```python
from build123d import *

# Parameters (mm, degrees)
F0_R     = 3
F1_DEPTH = 5
F2_R     = 3
F3_DEPTH = 3.5


with BuildPart() as f1:
    # F0 (on Top) → F1 (new body)
    with BuildSketch(Plane.XY):
        with BuildLine():
            ThreePointArc((-6.4258986346, 6.3014146616), (-5.2900672706, 7.2811529494), (-4.0072895936, 8.0586369886))
            ThreePointArc((-4.0072895936, 8.0586369886), (-6.1717451491, 8.4946784409), (-6.4258986346, 6.3014146616))
        make_face()
        with BuildLine():
            ThreePointArc((-1.4947825929, 8.875), (0, 9), (1.4947825929, 8.875))
            ThreePointArc((1.4947825929, 8.875), (1.4986950806, 8.937445581), (1.5, 9))
            ThreePointArc((1.5, 9), (-0.062554419, 10.4986950806), (-1.4947825929, 8.875))
        make_face()
        with BuildLine():
            ThreePointArc((4.0072895936, 8.0586369886), (5.2900672706, 7.2811529494), (6.4258986346, 6.3014146616))
            ThreePointArc((6.4258986346, 6.3014146616), (6.6960806145, 6.7585379123), (6.7900672706, 7.2811529494))
            ThreePointArc((6.7900672706, 7.2811529494), (5.6936967321, 8.7258270503), (4.0072895936, 8.0586369886))
        make_face()
        with BuildLine():
            ThreePointArc((7.978713358, 4.1641485505), (8.5595086467, 2.7811529494), (8.9025398062, 1.3209030997))
            ThreePointArc((8.9025398062, 1.3209030997), (9.7352098713, 1.8496344953), (10.0595086467, 2.7811529494))
            ThreePointArc((10.0595086467, 2.7811529494), (9.3898119247, 4.0303913039), (7.978713358, 4.1641485505))
        make_face()
        with BuildLine():
            ThreePointArc((10.0595086467, -2.7811529494), (9.7352098713, -1.8496344953), (8.9025398062, -1.3209030997))
            ThreePointArc((8.9025398062, -1.3209030997), (8.5595086467, -2.7811529494), (7.978713358, -4.1641485505))
            ThreePointArc((7.978713358, -4.1641485505), (9.3898119247, -4.0303913039), (10.0595086467, -2.7811529494))
        make_face()
        with BuildLine():
            ThreePointArc((6.7900672706, -7.2811529494), (6.6960806145, -6.7585379123), (6.4258986346, -6.3014146616))
            ThreePointArc((6.4258986346, -6.3014146616), (5.2900672706, -7.2811529494), (4.0072895936, -8.0586369886))
            ThreePointArc((4.0072895936, -8.0586369886), (5.6936967321, -8.7258270503), (6.7900672706, -7.2811529494))
        make_face()
        with BuildLine():
            ThreePointArc((1.5, -9), (1.4986950806, -8.937445581), (1.4947825929, -8.875))
            ThreePointArc((1.4947825929, -8.875), (0, -9), (-1.4947825929, -8.875))
            ThreePointArc((-1.4947825929, -8.875), (-0.062554419, -10.4986950806), (1.5, -9))
        make_face()
        with BuildLine():
            ThreePointArc((-6.4258986346, -6.3014146616), (-6.1717451491, -8.4946784409), (-4.0072895936, -8.0586369886))
            ThreePointArc((-4.0072895936, -8.0586369886), (-5.2900672706, -7.2811529494), (-6.4258986346, -6.3014146616))
        make_face()
        with BuildLine():
            ThreePointArc((-8.9025398062, -1.3209030997), (-9.9860934211, -3.2446784409), (-7.978713358, -4.1641485505))
            ThreePointArc((-7.978713358, -4.1641485505), (-8.5595086467, -2.7811529494), (-8.9025398062, -1.3209030997))
        make_face()
        with BuildLine():
            ThreePointArc((-8.9025398062, 1.3209030997), (-8.5595086467, 2.7811529494), (-7.978713358, 4.1641485505))
            ThreePointArc((-7.978713358, 4.1641485505), (-9.9860934211, 3.2446784409), (-8.9025398062, 1.3209030997))
        make_face()
        with BuildLine():
            ThreePointArc((8.9025398062, -1.3209030997), (8.9756018811, -0.6622468362), (9, 0))
            ThreePointArc((9, 0), (8.9756018811, 0.6622468362), (8.9025398062, 1.3209030997))
            ThreePointArc((8.9025398062, 1.3209030997), (7.1329238722, 2.3176274578), (7.978713358, 4.1641485505))
            ThreePointArc((7.978713358, 4.1641485505), (7.2811529494, 5.2900672706), (6.4258986346, 6.3014146616))
            ThreePointArc((6.4258986346, 6.3014146616), (4.4083893922, 6.0676274578), (4.0072895936, 8.0586369886))
            ThreePointArc((4.0072895936, 8.0586369886), (2.7811529494, 8.5595086467), (1.4947825929, 8.875))
            ThreePointArc((1.4947825929, 8.875), (0, 7.5), (-1.4947825929, 8.875))
            ThreePointArc((-1.4947825929, 8.875), (-2.7811529494, 8.5595086467), (-4.0072895936, 8.0586369886))
            ThreePointArc((-4.0072895936, 8.0586369886), (-3.8453931697, 7.6847824109), (-3.7900672706, 7.2811529494))
            ThreePointArc((-3.7900672706, 7.2811529494), (-4.7674522335, 5.8751396056), (-6.4258986346, 6.3014146616))
            ThreePointArc((-6.4258986346, 6.3014146616), (-7.2811529494, 5.2900672706), (-7.978713358, 4.1641485505))
            ThreePointArc((-7.978713358, 4.1641485505), (-7.3102702921, 3.6114562274), (-7.0595086467, 2.7811529494))
            ThreePointArc((-7.0595086467, 2.7811529494), (-7.6279901926, 1.6054517247), (-8.9025398062, 1.3209030997))
            ThreePointArc((-8.9025398062, 1.3209030997), (-9, 0), (-8.9025398062, -1.3209030997))
            ThreePointArc((-8.9025398062, -1.3209030997), (-7.6279901926, -1.6054517247), (-7.0595086467, -2.7811529494))
            ThreePointArc((-7.0595086467, -2.7811529494), (-7.3102702921, -3.6114562274), (-7.978713358, -4.1641485505))
            ThreePointArc((-7.978713358, -4.1641485505), (-7.2811529494, -5.2900672706), (-6.4258986346, -6.3014146616))
            ThreePointArc((-6.4258986346, -6.3014146616), (-4.7674522335, -5.8751396056), (-3.7900672706, -7.2811529494))
            ThreePointArc((-3.7900672706, -7.2811529494), (-3.8453931697, -7.6847824109), (-4.0072895936, -8.0586369886))
            ThreePointArc((-4.0072895936, -8.0586369886), (-2.7811529494, -8.5595086467), (-1.4947825929, -8.875))
            ThreePointArc((-1.4947825929, -8.875), (0, -7.5), (1.4947825929, -8.875))
            ThreePointArc((1.4947825929, -8.875), (2.7811529494, -8.5595086467), (4.0072895936, -8.0586369886))
            ThreePointArc((4.0072895936, -8.0586369886), (4.4083893922, -6.0676274578), (6.4258986346, -6.3014146616))
            ThreePointArc((6.4258986346, -6.3014146616), (7.2811529494, -5.2900672706), (7.978713358, -4.1641485505))
            ThreePointArc((7.978713358, -4.1641485505), (7.1329238722, -2.3176274578), (8.9025398062, -1.3209030997))
        make_face()
        Circle(F0_R, mode=Mode.SUBTRACT)
        with BuildLine():
            ThreePointArc((-7.0595086467, 2.7811529494), (-7.3102702921, 3.6114562274), (-7.978713358, 4.1641485505))
            ThreePointArc((-7.978713358, 4.1641485505), (-8.5595086467, 2.7811529494), (-8.9025398062, 1.3209030997))
            ThreePointArc((-8.9025398062, 1.3209030997), (-7.6279901926, 1.6054517247), (-7.0595086467, 2.7811529494))
        make_face()
        with BuildLine():
            ThreePointArc((-3.7900672706, 7.2811529494), (-3.8453931697, 7.6847824109), (-4.0072895936, 8.0586369886))
            ThreePointArc((-4.0072895936, 8.0586369886), (-5.2900672706, 7.2811529494), (-6.4258986346, 6.3014146616))
            ThreePointArc((-6.4258986346, 6.3014146616), (-4.7674522335, 5.8751396056), (-3.7900672706, 7.2811529494))
        make_face()
        with BuildLine():
            ThreePointArc((-1.4947825929, 8.875), (0, 7.5), (1.4947825929, 8.875))
            ThreePointArc((1.4947825929, 8.875), (0, 9), (-1.4947825929, 8.875))
        make_face()
        with BuildLine():
            ThreePointArc((4.0072895936, 8.0586369886), (4.4083893922, 6.0676274578), (6.4258986346, 6.3014146616))
            ThreePointArc((6.4258986346, 6.3014146616), (5.2900672706, 7.2811529494), (4.0072895936, 8.0586369886))
        make_face()
        with BuildLine():
            ThreePointArc((7.978713358, 4.1641485505), (7.1329238722, 2.3176274578), (8.9025398062, 1.3209030997))
            ThreePointArc((8.9025398062, 1.3209030997), (8.5595086467, 2.7811529494), (7.978713358, 4.1641485505))
        make_face()
        with BuildLine():
            ThreePointArc((7.978713358, -4.1641485505), (8.5595086467, -2.7811529494), (8.9025398062, -1.3209030997))
            ThreePointArc((8.9025398062, -1.3209030997), (7.1329238722, -2.3176274578), (7.978713358, -4.1641485505))
        make_face()
        with BuildLine():
            ThreePointArc((4.0072895936, -8.0586369886), (5.2900672706, -7.2811529494), (6.4258986346, -6.3014146616))
            ThreePointArc((6.4258986346, -6.3014146616), (4.4083893922, -6.0676274578), (4.0072895936, -8.0586369886))
        make_face()
        with BuildLine():
            ThreePointArc((-1.4947825929, -8.875), (0, -9), (1.4947825929, -8.875))
            ThreePointArc((1.4947825929, -8.875), (0, -7.5), (-1.4947825929, -8.875))
        make_face()
        Circle(F0_R)
        with BuildLine():
            ThreePointArc((-6.4258986346, -6.3014146616), (-5.2900672706, -7.2811529494), (-4.0072895936, -8.0586369886))
            ThreePointArc((-4.0072895936, -8.0586369886), (-3.8453931697, -7.6847824109), (-3.7900672706, -7.2811529494))
            ThreePointArc((-3.7900672706, -7.2811529494), (-4.7674522335, -5.8751396056), (-6.4258986346, -6.3014146616))
        make_face()
        with BuildLine():
            ThreePointArc((-8.9025398062, -1.3209030997), (-8.5595086467, -2.7811529494), (-7.978713358, -4.1641485505))
            ThreePointArc((-7.978713358, -4.1641485505), (-7.3102702921, -3.6114562274), (-7.0595086467, -2.7811529494))
            ThreePointArc((-7.0595086467, -2.7811529494), (-7.6279901926, -1.6054517247), (-8.9025398062, -1.3209030997))
        make_face()
    extrude(amount=F1_DEPTH)

    # F2 (on face) → F3 (cut)
    with BuildSketch(Plane.XY.offset(5)):
        Circle(F2_R)
    extrude(amount=-F3_DEPTH, mode=Mode.SUBTRACT)


solid = f1.part
```
The model under review builds one solid part; all positions refer to its coordinate system, in mm. A direction names the side the tool comes from. Give positions to 0.01 mm unless a question says otherwise; leave off trailing zeros. Write each loop counter-clockwise with the first axis right and the second up, starting at its lowest first coordinate (ties: lowest second). Pieces come first, ordered by that corner, then holes. Notation, with made-up numbers: (23.5, 81.5) - (69.5, 81.5) arc R22 cw to (69.5, 104.5) - close; hole circle Ø5 at (-32.75, 70). An arc over 180 degrees is marked (long way). Answer in a Markdown table with one row per item. Add a question column.
1. Tool access review of faces 1 (the cylindrical face through (2.763, -8.565, 2.465)), 2 (the cylindrical face through (-6.2, -8.474, 2.465)), 3 (the flat face through (2.1, 2.5, 5)), 4 (the flat face through (0, 0, 1.5)), 5 (the cylindrical face through (-2.763, 8.565, 2.465)): name each direction out of +Z, -Z, +X, -X, +Y, -Y from which nothing blocks a thin tool from reaching the whole face with its end or side.
2. We need section D-D on y = 5. Write out the cut boundary in (x, z), then the cut area to 3 significant figures.
3. Draft analysis for pull direction X (two halves, no side actions). For faces 6 (the cylindrical face through (-9, 0, 2)), 7 (the cylindrical face through (-2.799, -8.554, 2.465)), 8 (the flat face through (0, 0, 0)), state which applies: +X half, -X half, draft (parallel to the pull), parting line (faces both ways), or undercut.
4. Wall thickness on line 1 along Y through (x, z) = (0, 3); line 2 along Y through (x, z) = (6.5, 2.2); line 3 along X through (y, z) = (8.25, 2.85): over which ranges is each line inside the solid? List them lowest first. Write a range as [from, to].
5. We need section C-C on z = 1.25. Write out the cut boundary in (x, y) (1 decimal).
6. Insertion check: P1, Ø1, axis at x = -3.5, z = 3.5, coming from the +Y side; P2, Ø3, axis at y = 5.5, z = 4, coming from the +X side. Each pin has a flat end and moves straight along its axis. Give the tip position at first contact, or say it passes through.
7. We need section B-B on x = 0. Write out the cut boundary in (y, z).
8. We need section A-A on z = 2.9. Write out the cut boundary in (x, y) (1 decimal).
Ans:
| question | item | result |
|---|---|---|
| 1 | face 1 | +Z, -Z, -Y |
| 1 | face 2 | +Z, -Z |
| 1 | face 3 | +Z, +X, -X, +Y, -Y |
| 1 | face 4 | +Z |
| 1 | face 5 | +Z, -Z, +Y |
| 2 | outline | (-7.48, 0) - (7.48, 0) - (7.48, 5) - (-7.48, 5) - close |
| 2 | area | 74.8 mm^2 |
| 3 | face 6 | -X half |
| 3 | face 7 | undercut |
| 3 | face 8 | draft |
| 4 | line 1 | y = [-10.5, -3], [3, 10.5] |
| 4 | line 2 | y = [-8.17, -6.39], [-6.22, 6.22], [6.39, 8.17] |
| 4 | line 3 | x = [-6.44, -4.14], [-3.6, 3.6], [4.14, 6.44] |
| 5 | outline | (-8.9, -1.3) arc R1.5 ccw (long way) to (-8, -4.2) arc R9 ccw to (-6.4, -6.3) arc R1.5 ccw (long way) to (-4, -8.1) arc R9 ccw to (-1.5, -8.9) arc R1.5 ccw (long way) to (1.5, -8.9) arc R9 ccw to (4, -8.1) arc R1.5 ccw (long way) to (6.4, -6.3) arc R9 ccw to (8, -4.2) arc R1.5 ccw (long way) to (8.9, -1.3) arc R9 ccw to (8.9, 1.3) arc R1.5 ccw (long way) to (8, 4.2) arc R9 ccw to (6.4, 6.3) arc R1.5 ccw (long way) to (4, 8.1) arc R9 ccw to (1.5, 8.9) arc R1.5 ccw (long way) to (-1.5, 8.9) arc R9 ccw to (-4, 8.1) arc R1.5 ccw (long way) to (-6.4, 6.3) arc R9 ccw to (-8, 4.2) arc R1.5 ccw (long way) to (-8.9, 1.3) arc R9 ccw to start |
| 6 | P1 | stops at y = 8.49 |
| 6 | P2 | stops at x = 9.43 |
| 7 | outline | (-10.5, 0) - (10.5, 0) - (10.5, 5) - (3, 5) - (3, 1.5) - (-3, 1.5) - (-3, 5) - (-10.5, 5) - close |
| 8 | outline | (-8.9, -1.3) arc R1.5 ccw (long way) to (-8, -4.2) arc R9 ccw to (-6.4, -6.3) arc R1.5 ccw (long way) to (-4, -8.1) arc R9 ccw to (-1.5, -8.9) arc R1.5 ccw (long way) to (1.5, -8.9) arc R9 ccw to (4, -8.1) arc R1.5 ccw (long way) to (6.4, -6.3) arc R9 ccw to (8, -4.2) arc R1.5 ccw (long way) to (8.9, -1.3) arc R9 ccw to (8.9, 1.3) arc R1.5 ccw (long way) to (8, 4.2) arc R9 ccw to (6.4, 6.3) arc R1.5 ccw (long way) to (4, 8.1) arc R9 ccw to (1.5, 8.9) arc R1.5 ccw (long way) to (-1.5, 8.9) arc R9 ccw to (-4, 8.1) arc R1.5 ccw (long way) to (-6.4, 6.3) arc R9 ccw to (-8, 4.2) arc R1.5 ccw (long way) to (-8.9, 1.3) arc R9 ccw to start; hole circle Ø6 at (0, 0) |
